Here's how the part is built. I have some questions about the finished solid (model axes, mm). A direction names the side the tool comes from. Round coordinates to 2 decimals unless told otherwise and drop trailing zeros. Loops run counter-clockwise (first coordinate to the right, second up) from the corner with the lowest first, then second, coordinate; pieces in that order, holes last. Notation, with made-up numbers: M 33.5,52.25 L 72.5,52.25 A27 ccw 72.5,77.25 Z; hole C 73,14 d5. An arc over 180 degrees is marked long. Answer as a JSON object with one key per item and string values.
from build123d import *

# Parameters (mm, degrees)
EXTRU_MINCE1_DEPTH      = 25
EXTRU_MINCE2_DEPTH      = 40
ENL_V_MAT_EXTRU_1_REACH = 129.475
ESQUISSE3_R             = 9
CHANFREIN1_SIZE         = 4
ESQUISSE4_R             = 2.375
EXTRUSION1_DEPTH        = 10
CHANFREIN2_SIZE         = 3
EXTRUSION2_DEPTH        = 3
D_GAGEMENT_M31_D        = 3.4
D_GAGEMENT_M31_DEPTH    = 15
D_GAGEMENT_M31_TIP      = 1.021463052


with BuildPart() as part:
    # Esquisse1 → Extru.-Mince1 (new, symmetric)
    with BuildSketch(Plane.XY):
        with BuildLine():
            Line((-170, 0), (-9, 0))
            ThreePointArc((-9, 0), (-2.636038969, 2.636038969), (0, 9))
            Line((0, 9), (0, 30))
            Line((0, 30), (-4, 30))
            Line((-4, 30), (-4, 9))
            ThreePointArc((-4, 9), (-5.464466094, 5.464466094), (-9, 4))
            Line((-9, 4), (-170, 4))
            Line((-170, 4), (-170, 0))
        make_face()
    extrude(amount=EXTRU_MINCE1_DEPTH, both=True)

    # Esquisse2 → Extru.-Mince2 (add)
    with BuildSketch(Plane(origin=(0, 4, 0), x_dir=(-1, 0, 0), z_dir=(0, 1, 0))):
        with BuildLine():
            Line((110, -21), (114, -21))
            ThreePointArc((114, -21), (118.242640687, -19.242640687), (120, -15))
            Line((120, -15), (120, 15))
            ThreePointArc((120, 15), (118.242640687, 19.242640687), (114, 21))
            Line((114, 21), (110, 21))
            Line((110, 21), (110, 18))
            Line((110, 18), (114, 18))
            ThreePointArc((114, 18), (116.121320344, 17.121320344), (117, 15))
            Line((117, 15), (117, -15))
            ThreePointArc((117, -15), (116.121320344, -17.121320344), (114, -18))
            Line((114, -18), (110, -18))
            Line((110, -18), (110, -21))
        make_face()
    extrude(amount=EXTRU_MINCE2_DEPTH)

    # Esquisse3 → Enlèv. mat.-Extru.1 (cut, up to next)
    with BuildSketch(Plane(origin=(-117, 0, 0), x_dir=(0, 0, -1), z_dir=(1, 0, 0)), mode=Mode.PRIVATE) as enl_v_mat_extru_1_sk1:
        with Locations((0, 26)):
            Circle(ESQUISSE3_R)
    enl_v_mat_extru_1_tool1 = extrude(enl_v_mat_extru_1_sk1.sketch, amount=-ENL_V_MAT_EXTRU_1_REACH, mode=Mode.PRIVATE) & part.part
    add(enl_v_mat_extru_1_tool1.solids().sort_by_distance((-117, 26, 0))[0], mode=Mode.SUBTRACT)

    # Chanfrein1
    chanfrein1_edges = [part.edges().sort_by_distance(p)[0] for p in [
        (-170, 2, 25),
        (-170, 2, -25),
        (-2, 30, 25),
        (-2, 30, -25),
    ]]
    chamfer(chanfrein1_edges, length=CHANFREIN1_SIZE)

    # Esquisse4 → Extrusion1 (cut)
    with BuildSketch(Plane(origin=(0, 0, 0), x_dir=(0, 0, -1), z_dir=(1, 0, 0))):
        with Locations((0, 23.5)):
            Circle(ESQUISSE4_R)
        with BuildLine():
            Line((1.313915472, 30), (-1.386084528, 30))
            Line((-1.386084528, 30), (-1.386084528, 25.428573224))
            ThreePointArc((-1.386084528, 25.428573224), (-0.043862657, 25.874594927), (1.313915472, 25.478446646))
            Line((1.313915472, 25.478446646), (1.313915472, 30))
        make_face()
    extrude(amount=-EXTRUSION1_DEPTH, mode=Mode.SUBTRACT)

    # Chanfrein2
    chanfrein2_edges = [part.edges().sort_by_distance(p)[0] for p in [
        (-2, 30, 1.386084528),
        (-2, 30, -1.313915472),
    ]]
    chamfer(chanfrein2_edges, length=CHANFREIN2_SIZE)

    # Esquisse5 → Extrusion2 (cut)
    with BuildSketch(Plane(origin=(-117, 0, 0), x_dir=(0, 0, -1), z_dir=(1, 0, 0))):
        with BuildLine():
            Line((5.79, 44), (-5.79, 44))
            Line((-5.79, 44), (-5.79, 32.890275756))
            ThreePointArc((-5.79, 32.890275756), (0, 35), (5.79, 32.890275756))
            Line((5.79, 32.890275756), (5.79, 44))
        make_face()
    extrude(amount=-EXTRUSION2_DEPTH, mode=Mode.SUBTRACT)

    # Dégagement M31
    with Locations(Plane(origin=(-155, 4, -10.224980601), x_dir=(0, 0, 1), z_dir=(0, 1, 0))):
        with Locations((0, 0), (21.5, 0)):
            Hole(D_GAGEMENT_M31_D / 2, depth=D_GAGEMENT_M31_DEPTH)
            with Locations((0, 0, -(D_GAGEMENT_M31_DEPTH + D_GAGEMENT_M31_TIP / 2))):  # 118° drill point
                Cone(0, D_GAGEMENT_M31_D / 2, D_GAGEMENT_M31_TIP, mode=Mode.SUBTRACT)


solid = part.part
Item 1: I want a section at A-A, the plane x = -155. Please give me the cut outline in (y, z).
Resolved:
{"outline": "M 0,-25 L 4,-25 L 4,-11.92 L 0,-11.92 Z; M 0,-8.52 L 4,-8.52 L 4,9.58 L 0,9.58 Z; M 0,12.98 L 4,12.98 L 4,25 L 0,25 Z"}
Item 2: I'm going to push flat-ended pins straight in: pin 1 Ø3 at (x, y) = (-112, 33) entering from -Z; pin 2 Ø1.2 at (x, z) = (-2.5, 16) entering from +Y; pin 3 Ø0.9 at (y, z) = (19, 19) entering from +X; pin 4 Ø1.5 at (x, z) = (-69.5, 19) entering from +Y. Where does each tip first touch, or does it pass through?
Resolved:
{"pin 1": "z = -21", "pin 2": "y = 30", "pin 3": "x = 0", "pin 4": "y = 4"}
Item 3: I want a section at B-B, the plane y = 12. Please give me the cut outline in (x, z).
Resolved:
{"outline": "M -120,-15 A6 ccw -114,-21 L -110,-21 L -110,-18 L -114,-18 A3 cw -117,-15 L -117,15 A3 cw -114,18 L -110,18 L -110,21 L -114,21 A6 ccw -120,15 Z; M -4,-25 L 0,-25 L 0,25 L -4,25 Z"}
Item 4: I want a section at D-D, the plane x = -98. Please give me the cut outline in (y, z), then the cut area to 3 significant figures.
Resolved:
{"outline": "M 0,-25 L 4,-25 L 4,25 L 0,25 Z", "area": "200 mm²"}
Item 5: On a 3-axis mill with a long thin cutter (end or side, diameter ignored), from which of +Z, -Z, +X, -X, +Y, -Y can I reach the whole of each face in a straight line? I mean faces 1 (the face through (-2, 30, -13)), 2 (the face through (-118, 39, 5.79)), 3 (the face through (-117, 15, 0)), 4 (the face through (-110, 24, 20)). Say none if no direction works.
Resolved:
{"face 1": "+Z, -Z, +X, +Y", "face 2": "+X, -X, +Y", "face 3": "+Y", "face 4": "+Z, -Z, +Y"}
Item 6: I want a section at C-C, the plane y = 23.5. Please give me the cut outline in (x, z) (3 decimals), then the cut area to 3 significant figures.
Resolved:
{"outline": "M -120,-15 A6 ccw -114,-21 L -110,-21 L -110,-18 L -114,-18 A3 cw -117,-15 L -117,-8.646 L -120,-8.646 Z; M -120,8.646 L -117,8.646 L -117,15 A3 cw -114,18 L -110,18 L -110,21 L -114,21 A6 ccw -120,15 Z; M -4,-25 L 0,-25 L 0,-2.375 L -4,-2.375 Z; M -4,2.375 L 0,2.375 L 0,25 L -4,25 Z", "area": "286 mm²"}
Item 7: If we mould it in two halves opening along X, with no side actions, what happens to faces 5 (the face through (-112, 24, -18)), 6 (the face through (-170, 2, 0)), 7 (the face through (-118, 38, -5.79))? For each: pulls with the +X half, pulls with the -X half, needs draft (parallel to the pull), parting line crosses it, or undercut.
Resolved:
{"face 5": "undercut", "face 6": "pulls with the -X half", "face 7": "needs draft"}
Item 8: Please list where these lines run through material, in increasing order: probe 1 along Z at (x, y) = (-155, 2.3); probe 2 along X at (y, z) = (20, -11); probe 3 along Z at (x, y) = (-2.9, 23.5) (3 decimals). Write a range as from..to.
Resolved:
{"probe 1": "-25..-11.92, -8.52..9.58, 12.98..25", "probe 2": "-120..-117, -4..0", "probe 3": "-25..-2.375, 2.375..25"}
